from build123d import *


with BuildPart() as part:
    # Barrer1: sweep along a path in Croquis1
    with BuildLine(Plane(origin=(0, 0, 0), x_dir=(0, 0, -1), z_dir=(1, 0, 0))) as barrer1_path:
        Line((227.787907193, 23.812098623), (35.35962877, 95.248394492))
        ThreePointArc((35.35962877, 95.248394492), (-101.6, 0), (35.35962877, -95.248394492))
        Line((35.35962877, -95.248394492), (227.787907193, -23.812098623))
        ThreePointArc((227.787907193, -23.812098623), (244.348, 0), (227.787907193, 23.812098623))
    # Croquis2 → Barrer1 (sweep)
    with BuildSketch(Plane.XY):
        Polygon((-6.35, 101.6), (6.35, 101.6), (3.172084892, 92.86875), (-3.172084892, 92.86875), align=None)
    sweep(path=barrer1_path.line)


solid = part.part
Here's how the part is built. I have some questions about the finished solid (model axes, mm). A direction names the side the tool comes from. Give positions to 0.01 mm unless a question says otherwise; leave off trailing zeros. Order: outer loops, then holes, each group sorted by start corner. A loop starts at its lowest first (then second) coordinate and runs counter-clockwise, first axis right, second up. Notation, with made-up numbers: (89, 45.25) -> (111, 45.25) arc R12 ccw to (111, 49.25) -> close; hole circle Ø8 at (71, 38.25). An arc over 180 degrees is marked (long way). One line per item, written item: value. Start each with the question number.
1. Will these pins go through, and if not, where does the flat tip stop? pin 1 Ø3 at (x, y) = (3, -32) entering from +Z; pin 2 Ø3 at (x, z) = (2, -18.5) entering from +Y; pin 3 Ø4 at (x, z) = (-1, -177) entering from -Y.
2. For faces 1 (the face through (0.044, -0.284, -235.614)), 2 (the face through (-0.089, -0.432, -244.344)), 3 (the face through (-4.78, 55.99, -128.73)), 4 (the face through (4.74, 55.88, -128.69)), 5 (the face through (0, -59, -133)), which set-ups out of +Z, -Z, +X, -X, +Y, -Y let a thin tool reach every point of the face, with its end or its side?
3. Imagine slicing it at A-A, the plane z = 0. List the corners of the cut face in (x, y) for me, plus the area to 3 significant figures.
4. We'd pull the mould along Z, two halves only. Please class faces 6 (the face through (0.09, 60.03, -130.23)), 7 (the face through (4.74, -54.88, -131.38)), 8 (the face through (-0.089, 2.74, 101.563)): released by +Z, released by -Z, zero draft, split by the parting line, or undercut.
5. I need wall thicknesses on probe 1 along Y at (x, z) = (-1, 0); probe 2 along Y at (x, z) = (-1.5, -17); probe 3 along X at (y, z) = (-79, 55). Which ranges of each line are inside material? Lowest first, please. Write a range as from..to.
6. Imagine slicing it at B-B, the plane y = 0. List the corners of the cut face in (x, z) for me.
Values follow:
1. pin 1: stops at z = 96.91
1. pin 2: stops at y = 100.17
1. pin 3: stops at y = -43.41
2. face 1: +X, -X
2. face 2: -Z, +X, -X
2. face 3: -X
2. face 4: +X
2. face 5: -Z, +X, -X, -Y
3. outline: (-6.35, -101.6) -> (6.35, -101.6) -> (3.17, -92.87) -> (-3.17, -92.87) -> close; (-6.35, 101.6) -> (-3.17, 92.87) -> (3.17, 92.87) -> (6.35, 101.6) -> close
3. area: 166 mm2
4. face 6: released by -Z
4. face 7: undercut
4. face 8: split by the parting line
5. probe 1: y = -101.6..-92.87, 92.87..101.6
5. probe 2: y = -100.17..-91.3, 91.3..100.17
5. probe 3: x = -4.41..4.41
6. outline: (-6.35, -244.35) -> (6.35, -244.35) -> (3.17, -235.62) -> (-3.17, -235.62) -> close; (-6.35, 101.6) -> (-3.17, 92.87) -> (3.17, 92.87) -> (6.35, 101.6) -> close
